Source: CAD feature listing. Evaluate the final solid. Frame: model axes, mm. A direction names the side the tool comes from. Give positions to 0.01 mm unless a question says otherwise; leave off trailing zeros. Order: outer loops, then holes, each group sorted by start corner. A loop starts at its lowest first (then second) coordinate and runs counter-clockwise, first axis right, second up. Notation, with made-up numbers: (-26, -24) - (21, -24) arc R20 ccw to (21, -11) - close; hole circle Ø6 at (-29.75, 48.25). An arc over 180 degrees is marked (long way). Use CSV: the item, a comma, the result in double quotes.
```python
from build123d import *

# Parameters (mm, degrees)
F0_W     = 18.25752
F0_H     = 6.19252
F1_DEPTH = 3.175
F2_W     = 1.27
F2_H     = 1.27
F3_DEPTH = 0.635
F5_W     = 0.762
F5_H     = 0.508
F6_DEPTH = 25.4
F7_R     = 0.254


with BuildPart() as f1:
    # F0 (on Top) → F1 (new body)
    with BuildSketch(Plane.XY):
        with Locations((-0.4847390454, 0.6100881006)):
            Rectangle(F0_W, F0_H)
    extrude(amount=F1_DEPTH)

    # F2 (on Top) → F3 (join)
    with BuildSketch(Plane.XY):
        with Locations((-7.6322990454, 4.3413481006)):
            Rectangle(F2_W, F2_H)
        with Locations((-5.2497790454, 4.3413481006)):
            Rectangle(F2_W, F2_H)
        with Locations((-2.8672590454, 4.3413481006)):
            Rectangle(F2_W, F2_H)
        with Locations((-0.4847390454, 4.3413481006)):
            Rectangle(F2_W, F2_H)
        with Locations((1.8977809546, 4.3413481006)):
            Rectangle(F2_W, F2_H)
        with Locations((4.2803009546, 4.3413481006)):
            Rectangle(F2_W, F2_H)
        with Locations((6.6628209546, 4.3413481006)):
            Rectangle(F2_W, F2_H)
        with Locations((-7.6322990454, -3.1211718994)):
            Rectangle(F2_W, F2_H)
        with Locations((-5.2497790454, -3.1211718994)):
            Rectangle(F2_W, F2_H)
        with Locations((-2.8672590454, -3.1211718994)):
            Rectangle(F2_W, F2_H)
        with Locations((-0.4847390454, -3.1211718994)):
            Rectangle(F2_W, F2_H)
        with Locations((1.8977809546, -3.1211718994)):
            Rectangle(F2_W, F2_H)
        with Locations((4.2803009546, -3.1211718994)):
            Rectangle(F2_W, F2_H)
        with Locations((6.6628209546, -3.1211718994)):
            Rectangle(F2_W, F2_H)
    extrude(amount=F3_DEPTH)

    # F5 (on face) → F6 (cut)
    with BuildSketch(Plane(origin=(-9.6134990454, 0, 0), x_dir=(0, -1, 0), z_dir=(-1, 0, 0))):
        with Locations((-3.3253481006, 2.921)):
            Rectangle(F5_W, F5_H)
        with Locations((2.1051718994, 2.921)):
            Rectangle(F5_W, F5_H)
    extrude(amount=-F6_DEPTH, mode=Mode.SUBTRACT)

    # F7
    f7_edges = [f1.edges().sort_by_distance(p)[0] for p in [
        (-0.484739, 3.706348, 2.667),
        (-0.484739, 2.944348, 3.175),
        (-0.484739, -1.724172, 3.175),
        (-0.484739, -2.486172, 2.667),
        (-9.613499, 0.610088, 3.175),
        (-9.613499, -1.724172, 2.921),
        (-9.613499, -2.105172, 2.667),
        (-9.613499, -2.486172, 1.3335),
        (-9.613499, 3.325348, 2.667),
        (-9.613499, 2.944348, 2.921),
        (-9.613499, 3.706348, 1.3335),
        (8.644021, -2.486172, 1.3335),
        (8.644021, -2.105172, 2.667),
        (8.644021, -1.724172, 2.921),
        (8.644021, 0.610088, 3.175),
        (8.644021, 2.944348, 2.921),
        (8.644021, 3.325348, 2.667),
        (8.644021, 3.706348, 1.3335),
    ]]
    fillet(f7_edges, radius=F7_R)


solid = f1.part
```
Item 1: First-contact query: pin 1 (0.5 mm diameter, centred on y = -3, z = 0.5, fed in from -X); pin 2 (0.5 mm diameter, centred on y = -3, z = 0, fed in from +X); pin 3 (1.4 mm diameter, centred on x = 4, y = -3, fed in from +Z). Flat tips, straight axial feed; report the tip coordinate or a pass-through.
Filled in:
pin 1,"stops at x = -8.27"
pin 2,"stops at x = 7.3"
pin 3,"stops at z = 2.66"
Item 2: Section A-A on z = 1.45. Return the cut outline in (x, y).
Filled in:
outline,"(-9.61, -2.23) arc R0.25 ccw to (-9.36, -2.49) - (8.39, -2.49) arc R0.25 ccw to (8.64, -2.23) - (8.64, 3.45) arc R0.25 ccw to (8.39, 3.71) - (-9.36, 3.71) arc R0.25 ccw to (-9.61, 3.45) - close"
Item 3: Material intervals for line 1 (Y direction, x = 4.5, z = 2.2); line 2 (X direction, y = 2, z = 2.95); line 3 (Z direction, x = -3, y = 3.75) (3 decimals), sorted ascending. Write a range as from..to.
Filled in:
line 1,"y = -2.49..3.71"
line 2,"x = -9.61..8.64"
line 3,"z = 0..0.635"
Item 4: Section C-C on x = 5.25. Return the cut outline in (y, z) (3 decimals).
Filled in:
outline,"(-2.486, 0) - (3.706, 0) - (3.706, 2.413) arc R0.254 ccw to (3.452, 2.667) - (2.944, 2.667) - (2.944, 2.921) arc R0.254 ccw to (2.69, 3.175) - (-1.47, 3.175) arc R0.254 ccw to (-1.724, 2.921) - (-1.724, 2.667) - (-2.232, 2.667) arc R0.254 ccw to (-2.486, 2.413) - close"
Item 5: Section B-B on x = -2.5. Return the cut outline in (y, z) (3 decimals), then the cut area to 3 significant figures.
Filled in:
outline,"(-3.756, 0) - (4.976, 0) - (4.976, 0.635) - (3.706, 0.635) - (3.706, 2.413) arc R0.254 ccw to (3.452, 2.667) - (2.944, 2.667) - (2.944, 2.921) arc R0.254 ccw to (2.69, 3.175) - (-1.47, 3.175) arc R0.254 ccw to (-1.724, 2.921) - (-1.724, 2.667) - (-2.232, 2.667) arc R0.254 ccw to (-2.486, 2.413) - (-2.486, 0.635) - (-3.756, 0.635) - close"
area,"20.4 mm2"
Item 6: Set-up query: faces 1 (the flat face through (-1, 1, 3.175)), 2 (the flat face through (-5, -3, 0.635)), 3 (the flat face through (-3, 4, 0.635)). Return all of +Z, -Z, +X, -X, +Y, -Y with unobstructed straight access to the full face (end or side cutting, diameter ignored); none if empty.
Filled in:
face 1,"+Z, +X, -X, +Y, -Y"
face 2,"+Z, +X, -X, -Y"
face 3,"+Z, +X, -X, +Y"
